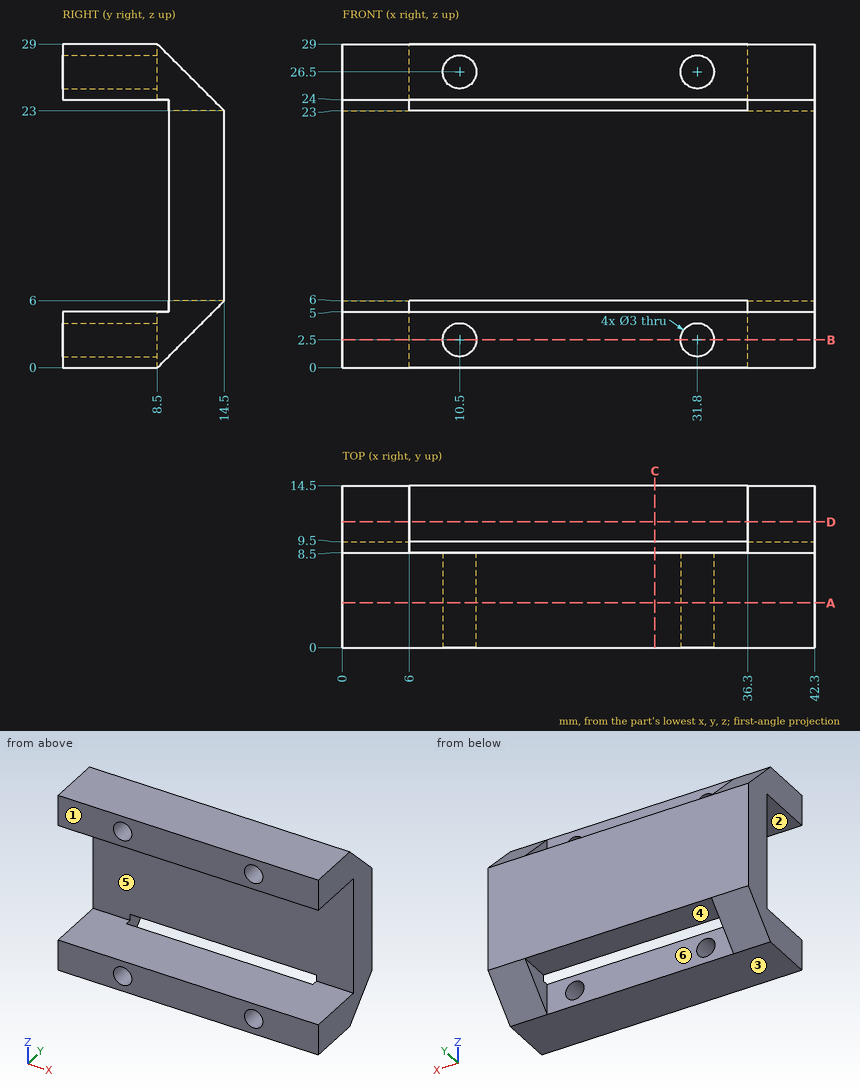
The drawing under review shows one solid part. Ordinate dimensions are in mm from its lowest x, y, z. A direction names the side the tool comes from. Round coordinates to 2 decimals unless told otherwise and drop trailing zeros. Loops run counter-clockwise (first coordinate to the right, second up) from the corner with the lowest first, then second, coordinate; pieces in that order, holes last.
Item 1: Mouldability with a two-part tool opening along Z and no side actions: class the marked faces 1, 2 and 3 as released by +Z, released by -Z, zero draft, split by the parting line, or undercut.
Determined:
face 1: zero draft
face 2: undercut
face 3: released by -Z
Item 2: For line 1 (Z direction, x = 31.8, y = 4.25); line 2 (Z direction, x = 4.5, y = 4.5); line 3 (X direction, y = 10.75, z = 5.5), list the stretches that pass through material, from the lowest coordinate up.
Determined:
line 1: z = 0 to 1, 4 to 5, 24 to 25, 28 to 29
line 2: z = 0 to 5, 24 to 29
line 3: x = 0 to 6, 36.3 to 42.3
Item 3: Clearance check with flat-ended pins moving along their axes: pin 1 Ø5.5 at (x, y) = (23.5, 11.5) entering from -Z; pin 2 Ø5.5 at (x, z) = (15, 3) entering from +Y; pin 3 Ø3 at (x, y) = (18.5, 11.5) entering from +Z. State where each tip first meets the part, or that it passes through.
Determined:
pin 1: stops at z = 6
pin 2: stops at y = 8.5
pin 3: stops at z = 23
Item 4: For the marked faces 4, 5 and 6, list the 3-axis set-ups (+Z, -Z, +X, -X, +Y, -Y) from which the entire face can be reached by the end or side of a thin tool; tool diameter is ignored.
Determined:
face 4: -Z, +Y, -Y
face 5: +X, -X, -Y
face 6: +Z, -Z, +Y
Item 5: Take a section at A-A (y = 4). Write out the cut boundary in (x, z), then the cut area to 3 significant figures.
Determined:
outline: (0, 0) - (42.3, 0) - (42.3, 5) - (0, 5) - close; (0, 24) - (42.3, 24) - (42.3, 29) - (0, 29) - close; hole circle Ø3 at (10.5, 2.5); hole circle Ø3 at (10.5, 26.5); hole circle Ø3 at (31.8, 2.5); hole circle Ø3 at (31.8, 26.5)
area: 395 mm2
Item 6: Take a section at D-D (y = 11.25). Write out the cut boundary in (x, z).
Determined:
outline: (0, 2.75) - (6, 2.75) - (6, 6) - (36.3, 6) - (36.3, 2.75) - (42.3, 2.75) - (42.3, 26.25) - (36.3, 26.25) - (36.3, 23) - (6, 23) - (6, 26.25) - (0, 26.25) - close
Item 7: Take a section at C-C (x = 28). Write out the cut boundary in (y, z), then the cut area to 3 significant figures.
Determined:
outline: (0, 0) - (8.5, 0) - (8.5, 5) - (0, 5) - close; (0, 24) - (8.5, 24) - (8.5, 29) - (0, 29) - close; (9.5, 6) - (14.5, 6) - (14.5, 23) - (9.5, 23) - close
area: 170 mm2
Item 8: Take a section at B-B (z = 2.5). Write out the cut boundary in (x, y).
Determined:
outline: (0, 0) - (9, 0) - (9, 8.5) - (6, 8.5) - (6, 11) - (0, 11) - close; (12, 0) - (30.3, 0) - (30.3, 8.5) - (12, 8.5) - close; (33.3, 0) - (42.3, 0) - (42.3, 11) - (36.3, 11) - (36.3, 8.5) - (33.3, 8.5) - close
